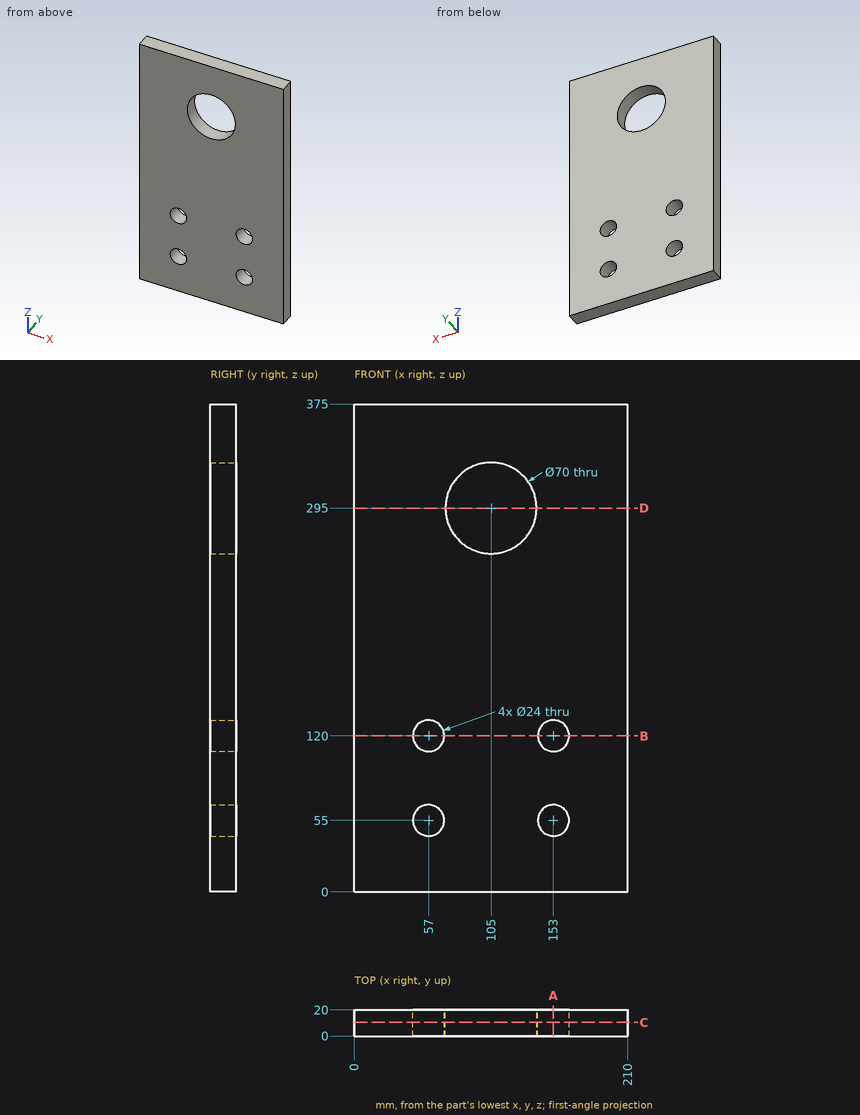
Verification items for this drawing (mm, ordinates from the low corner). Coordinates: 2 decimals unless noted, no trailing zeros. Loops run counter-clockwise (first coordinate to the right, second up) from the corner with the lowest first, then second, coordinate; pieces in that order, holes last. Notation, with made-up numbers: (-27.5, -35) -> (-4.5, -35) arc R27 cw to (-4.5, -12) -> close; hole circle Ø4 at (25.25, 66). An arc over 180 degrees is marked (long way). Put each result on its own line as item: value.
1. Section check A-A, the plane x = 153. Record the boundary of the cut face in (y, z).
Result set:
outline: (0, 0) -> (20, 0) -> (20, 43) -> (0, 43) -> close; (0, 67) -> (20, 67) -> (20, 108) -> (0, 108) -> close; (0, 132) -> (20, 132) -> (20, 375) -> (0, 375) -> close
2. Section check C-C, the plane y = 10.5. Record the boundary of the cut face in (x, z).
Result set:
outline: (0, 0) -> (210, 0) -> (210, 375) -> (0, 375) -> close; hole circle Ø24 at (57, 55); hole circle Ø24 at (57, 120); hole circle Ø70 at (105, 295); hole circle Ø24 at (153, 55); hole circle Ø24 at (153, 120)
3. Thickness scan on line 1 (Z direction, x = 57, y = 10); line 2 (X direction, y = 13, z = 114); line 3 (X direction, y = 13, z = 45.5). Record the ranges inside material, lowest first.
Result set:
line 1: z = 0 to 43, 67 to 108, 132 to 375
line 2: x = 0 to 46.61, 67.39 to 142.61, 163.39 to 210
line 3: x = 0 to 49.67, 64.33 to 145.67, 160.33 to 210
4. Section check D-D, the plane z = 295. Record the boundary of the cut face in (x, y), then the cut area to 3 significant figures.
Result set:
outline: (0, 0) -> (70, 0) -> (70, 20) -> (0, 20) -> close; (140, 0) -> (210, 0) -> (210, 20) -> (140, 20) -> close
area: 2,800 mm^2
5. Section check B-B, the plane z = 120. Record the boundary of the cut face in (x, y), then the cut area to 3 significant figures.
Result set:
outline: (0, 0) -> (45, 0) -> (45, 20) -> (0, 20) -> close; (69, 0) -> (141, 0) -> (141, 20) -> (69, 20) -> close; (165, 0) -> (210, 0) -> (210, 20) -> (165, 20) -> close
area: 3,240 mm^2
